```python
from build123d import *

# Parameters (mm, degrees)
SKETCH_1_W                   = 30
SKETCH_1_H                   = 195
EXTRUDE_1_DEPTH              = 5
SKETCH_2_W                   = 4
SKETCH_2_H                   = 195
SKETCH_2_W_2                 = 3
EXTRUDE_2_DEPTH              = 10
SKETCH_3_W                   = 4
SKETCH_3_H                   = 3
CUT_EXTRUDE_1_DEPTH          = 197.150452459
HOLE_WIZARD_M5_1_D           = 5.5
HOLE_WIZARD_M5_1_CBORE_D     = 11
HOLE_WIZARD_M5_1_CBORE_DEPTH = 3
SKETCH_7_W                   = 6.1
SKETCH_7_H                   = 120
EXTRUDE_3_DEPTH              = 6


with BuildPart() as part:
    # 스케치1 → 보스-돌출1 (new body)
    with BuildSketch(Plane(origin=(0, 0, 0), x_dir=(1, 0, 0), z_dir=(0, 1, 0))):
        Rectangle(SKETCH_1_W, SKETCH_1_H)
    extrude(amount=EXTRUDE_1_DEPTH)

    # 스케치2 → 보스-돌출2 (add)
    with BuildSketch(Plane(origin=(0, 5, 0), x_dir=(1, 0, 0), z_dir=(0, 1, 0))):
        with Locations((-13, 0)):
            Rectangle(SKETCH_2_W, SKETCH_2_H)
        with Locations((13.5, 0)):
            Rectangle(SKETCH_2_W_2, SKETCH_2_H)
    extrude(amount=EXTRUDE_2_DEPTH)

    # 스케치3 → 컷-돌출1 (cut, through all)
    with BuildSketch(Plane.XY.offset(97.5)):
        with Locations((-13, 13.5)):
            Rectangle(SKETCH_3_W, SKETCH_3_H)
        Polygon((12, 5), (12, 15), (13.5, 15), align=None)
    extrude(amount=-CUT_EXTRUDE_1_DEPTH, mode=Mode.SUBTRACT)

    # M5 소켓 머리 캡 나사용 카운터보어1 (through all)
    with Locations(Plane(origin=(0, 5, 0), x_dir=(1, 0, 0), z_dir=(0, 1, 0))):
        with Locations((0, -82.5), (0, 82.5)):
            CounterBoreHole(HOLE_WIZARD_M5_1_D / 2, HOLE_WIZARD_M5_1_CBORE_D / 2, HOLE_WIZARD_M5_1_CBORE_DEPTH)

    # 스케치7 → 보스-돌출3 (add)
    with BuildSketch(Plane.XZ):
        Rectangle(SKETCH_7_W, SKETCH_7_H)
    extrude(amount=EXTRUDE_3_DEPTH)


solid = part.part
```
CAD build for the part. Positions are in the model's coordinates, mm. A direction names the side the tool comes from. Give positions to 0.01 mm unless a question says otherwise; leave off trailing zeros. Loops run counter-clockwise (first coordinate to the right, second up) from the corner with the lowest first, then second, coordinate; pieces in that order, holes last. Notation, with made-up numbers: (48, 19) -> (72, 19) arc R24 cw to (72, 43) -> close; hole circle Ø2 at (-3.75, 49). An arc over 180 degrees is marked (long way). Use a Markdown table: item, result.
1. Mould opens along Z. For faces 1 (the cylindrical face through (0.596, 0.986, -79.815)), 2 (the flat face through (0, -3, -60)), 3 (the flat face through (-11, 8, 1)) say: pulls with the +Z half, pulls with the -Z half, needs draft (parallel to the pull), parting line crosses it, or undercut.
Check result:
| item | result |
|---|---|
| face 1 | undercut |
| face 2 | pulls with the -Z half |
| face 3 | needs draft |
2. Slice it at C-C (x = 0). List the corners of the cut face in (y, z), plus the area to 3 significant figures.
Check result:
| item | result |
|---|---|
| outline | (-6, -60) -> (0, -60) -> (0, -79.75) -> (2, -79.75) -> (2, -77) -> (5, -77) -> (5, 77) -> (2, 77) -> (2, 79.75) -> (0, 79.75) -> (0, 60) -> (-6, 60) -> close; (0, -97.5) -> (5, -97.5) -> (5, -88) -> (2, -88) -> (2, -85.25) -> (0, -85.25) -> close; (0, 85.25) -> (2, 85.25) -> (2, 88) -> (5, 88) -> (5, 97.5) -> (0, 97.5) -> close |
| area | 1,610 mm^2 |
3. Flat gauge pins, fed straight in: pin 1 (11.5 mm diameter, centred on x = -3, z = 44.5, fed in from +Y); pin 2 (5 mm diameter, centred on x = 11.5, z = -23, fed in from +Y); pin 3 (17.5 mm diameter, centred on x = 0, z = 82.5, fed in from -Y); pin 4 (3.5 mm diameter, centred on x = 0, z = -82.5, fed in from -Y). Where does each tip first touch, or does it go through?
Check result:
| item | result |
|---|---|
| pin 1 | stops at y = 5 |
| pin 2 | stops at y = 15 |
| pin 3 | stops at y = 0 |
| pin 4 | passes through |
4. Slice it at A-A (y = 7). List the corners of the cut face in (x, z).
Check result:
| item | result |
|---|---|
| outline | (-15, -97.5) -> (-11, -97.5) -> (-11, 97.5) -> (-15, 97.5) -> close; (12.3, -97.5) -> (15, -97.5) -> (15, 97.5) -> (12.3, 97.5) -> close |
5. Slice it at B-B (z = -82.5). List the corners of the cut face in (x, y).
Check result:
| item | result |
|---|---|
| outline | (-15, 0) -> (-2.75, 0) -> (-2.75, 2) -> (-5.5, 2) -> (-5.5, 5) -> (-11, 5) -> (-11, 12) -> (-15, 12) -> close; (2.75, 0) -> (15, 0) -> (15, 15) -> (13.5, 15) -> (12, 5) -> (5.5, 5) -> (5.5, 2) -> (2.75, 2) -> close |
6. Which spindle directions (+Z, -Z, +X, -X, +Y, -Y) get a long thin tool onto all of the face, cutting with end or side? Do faces 4 (the cylindrical face through (-0.716, 3.521, 77.047)), 5 (the flat face through (-3.05, -3, -1)), 6 (the flat face through (0, -3, 60)), 7 (the flat face through (-13, 12, 1)), 8 (the flat face through (0, 5, -1)). Say none if no direction does.
Check result:
| item | result |
|---|---|
| face 4 | +Y |
| face 5 | +Z, -Z, -X, -Y |
| face 6 | +Z, +X, -X, -Y |
| face 7 | +Z, -Z, -X, +Y |
| face 8 | +Z, -Z, +Y |
7. Wall check: L1, parallel to Z at x = 0, y = 0.75; L2, parallel to Z at x = 0, y = 3.9; L3, parallel to X at y = 1.5, z = 82.5. Give the ranges that are in metal, low to high. Write a range as [from, to].
Check result:
| item | result |
|---|---|
| L1 | z = [-97.5, -85.25], [-79.75, 79.75], [85.25, 97.5] |
| L2 | z = [-97.5, -88], [-77, 77], [88, 97.5] |
| L3 | x = [-15, -2.75], [2.75, 15] |
8. Slice it at D-D (z = -57). List the corners of the cut face in (x, y).
Check result:
| item | result |
|---|---|
| outline | (-15, 0) -> (-3.05, 0) -> (-3.05, -6) -> (3.05, -6) -> (3.05, 0) -> (15, 0) -> (15, 15) -> (13.5, 15) -> (12, 5) -> (-11, 5) -> (-11, 12) -> (-15, 12) -> close |
